Geometry check sheet. Reference: the model listing, model coordinates, mm. Face numbers are marked on the shaded views. A direction names the side the tool comes from. Coordinates: 2 decimals unless noted, no trailing zeros. Order: outer loops, then holes, each group sorted by start corner. A loop starts at its lowest first (then second) coordinate and runs counter-clockwise, first axis right, second up. Notation, with made-up numbers: (48, 36.25) - (71, 36.25) arc R12 ccw to (71, 56.25) - close; hole circle Ø2 at (-18.75, -34). An arc over 180 degrees is marked (long way). Return JSON: item names as keys, results as strings. Group by question number.
Item 1: Section check B-B on y = 52.5. Enter the section's corners in (x, z) (3 decimals).
Item 2: Section check A-A on z = 2. Enter the section's corners in (x, y) (3 decimals).
Item 3: Tool access check on the marked faces 1, 2, 3, 4 and 5. Record the directions out of +Z, -Z, +X, -X, +Y, -Y that give a thin tool (end or side, any length) a straight path to the whole face; none if there is none.
Item 4: Gauge pin test, flat ends, axial feed: pin 1 (10.5 mm diameter, centred on y = -21.5, z = 20, fed in from -X) (3 decimals); pin 2 (15.5 mm diameter, centred on x = 96.5, y = 9, fed in from -Z); pin 3 (1.5 mm diameter, centred on x = 0.5, y = -33, fed in from +Z) (3 decimals); pin 4 (8 mm diameter, centred on x = 74.5, y = 24.5, fed in from +Z) (3 decimals). Record the tip position at first contact, or that the pin passes through.
Item 5: Scan lines: probe 1 along X at (y, z) = (51, 4) (3 decimals); probe 2 along Z at (x, y) = (-18, -17) (3 decimals); probe 3 along Y at (x, z) = (75.5, 50). Record each from-to range of solid material in increasing order.
Item 6: Draft check along X on the marked faces 6, 7, 8 and 9. Enter one of: pulls with the +X half, pulls with the -X half, needs draft (parallel to the pull), parting line crosses it, or undercut.
Item 7: Section check C-C on x = 85. Enter the section's corners in (y, z) (3 decimals), then the cut area to 3 significant figures.
from build123d import *

# Parameters (mm, degrees)
F1_DEPTH = 63.5
F0_W     = 25.0189637039
F0_H     = 19.05
F2_DEPTH = 25.4
F3_DEPTH = 15.875
F5_R     = 6.35


with BuildPart() as f1:
    # F0 (on Front) → F1 (new body, symmetric)
    with BuildSketch(Plane.XZ):
        Polygon((22.225, 9.525), (-41.275, 9.525), (-41.275, -9.525), (41.275, -9.525), (41.275, 9.525), align=None)
    extrude(amount=F1_DEPTH, both=True)

    # F0 (on Front) → F2 (join, symmetric)
    with BuildSketch(Plane.XZ):
        with BuildLine():
            Line((22.225, 27.0002), (22.225, 9.525))
            Line((22.225, 9.525), (41.275, 9.525))
            Line((41.275, 9.525), (41.275, 27.0002))
            ThreePointArc((41.275, 27.0002), (45.9246798487, 38.2255201513), (57.15, 42.8752))
            Line((57.15, 42.8752), (60.325, 42.8752))
            Line((60.325, 42.8752), (60.325, 61.9252))
            Line((60.325, 61.9252), (57.15, 61.9252))
            ThreePointArc((57.15, 61.9252), (32.4542956671, 51.6959043329), (22.225, 27.0002))
        make_face()
        with Locations((72.8344818519, 52.4002)):
            Rectangle(F0_W, F0_H)
    extrude(amount=F2_DEPTH, both=True)

    # F0 (on Front) → F3 (join)
    with BuildSketch(Plane.XZ):
        with BuildLine():
            add(Edge.make_bspline(
                [(57.15, 61.9252), (-3.7140410859, 62.1167458594), (-38.0423441529, 46.5129725635), (-41.275, 9.525)],
                knots=[0, 0, 0, 0, 111.5045361635, 111.5045361635, 111.5045361635, 111.5045361635], degree=3))
            Line((-41.275, 9.525), (22.225, 9.525))
            Line((22.225, 9.525), (22.225, 27.0002))
            ThreePointArc((22.225, 27.0002), (32.4542956671, 51.6959043329), (57.15, 61.9252))
        make_face()
    extrude(amount=F3_DEPTH)

    # F0 (on Front) → F4 (revolve)
    with BuildSketch(Plane.XZ):
        Polygon((85.3439637039, 66.675), (85.3439637039, 61.9252), (85.3439637039, 42.8752), (85.3439637039, 38.1), (111.125, 38.1), (111.125, 66.675), align=None)
    revolve(axis=Axis((85.3439637039, 0, 52.3875), (0, 0, -1)))

    # F5
    f5_edges = [f1.edges().sort_by_distance(p)[0] for p in [
        (-41.275, 63.5, 0),
        (41.275, 63.5, 0),
        (41.275, -63.5, 0),
        (-41.275, -63.5, 0),
    ]]
    fillet(f5_edges, radius=F5_R)


solid = f1.part
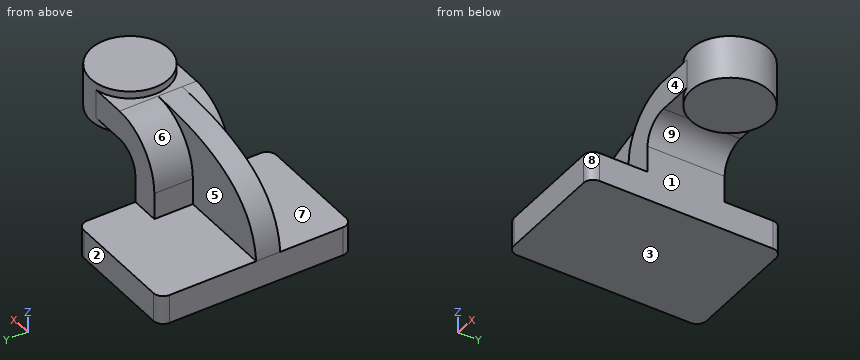
Computed:
{
 "1": {"outline": "(-41.275, -9.525) - (41.275, -9.525) - (41.275, 9.525) - (-41.275, 9.525) - close"},
 "2": {"outline": "(-41.275, -57.15) arc R6.35 ccw to (-34.925, -63.5) - (34.925, -63.5) arc R6.35 ccw to (41.275, -57.15) - (41.275, 57.15) arc R6.35 ccw to (34.925, 63.5) - (-34.925, 63.5) arc R6.35 ccw to (-41.275, 57.15) - close"},
 "3": {"face 1": "-Z, +X, +Y, -Y", "face 2": "+Z, -Z, +X, -X, +Y", "face 3": "-Z, +X, -X, +Y, -Y", "face 4": "+Z, -X, -Y", "face 5": "+Z, -X, +Y"},
 "4": {"pin 1": "stops at x = 22.225", "pin 2": "stops at z = 38.1", "pin 3": "stops at z = 9.525", "pin 4": "stops at z = 66.675"},
 "5": {"probe 1": "x = -41.275 to 41.275", "probe 2": "z = -9.525 to 9.525", "probe 3": "y = -25.4 to 25.4"},
 "6": {"face 6": "pulls with the -X half", "face 7": "needs draft", "face 8": "pulls with the +X half", "face 9": "undercut"},
 "7": {"outline": "(-25.779, 38.1) - (25.779, 38.1) - (25.779, 66.675) - (-25.779, 66.675) - close", "area": "1,470 mm²"}
}
